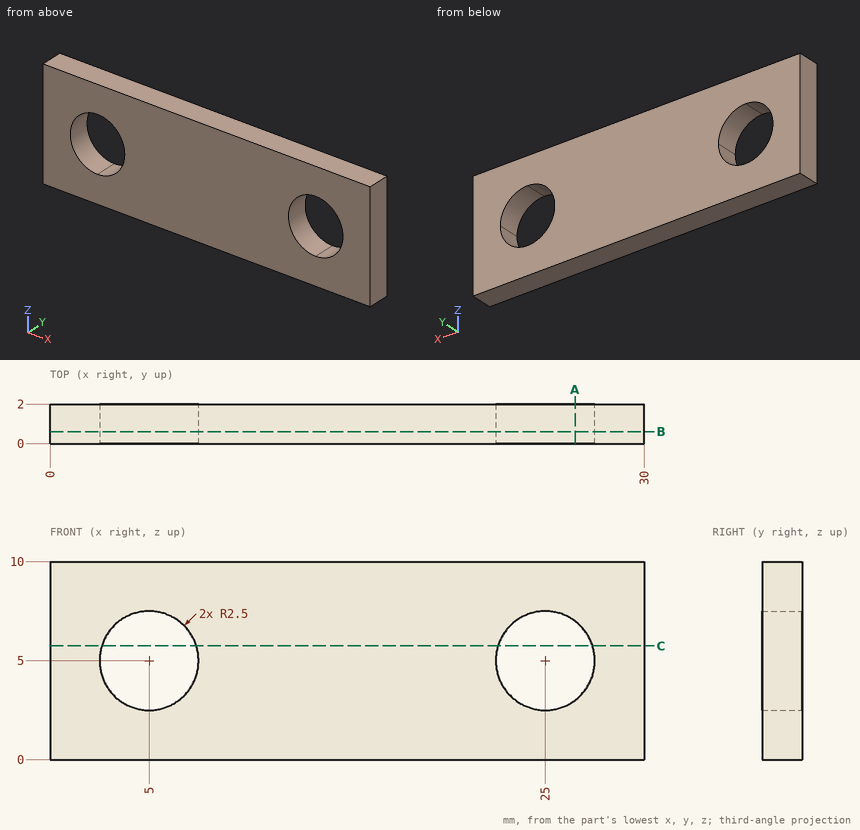
Answer from the drawing. Dimensions are ordinates in mm from the lowest x, y and z of the part. Give positions to 0.01 mm unless a question says otherwise; leave off trailing zeros. Loops run counter-clockwise (first coordinate to the right, second up) from the corner with the lowest first, then second, coordinate; pieces in that order, holes last.
Item 1: The part is cut by section A-A (x = 26.5). Write down the section's boundary in (y, z).
Item 2: The part is cut by section B-B (y = 0.6). Write down the section's boundary in (x, z).
Item 3: Find the intervals of material crossed by line 1 along X through (y, z) = (1.5, 6); line 2 along X through (y, z) = (0.25, 3.5); line 3 along Z through (x, y) = (4.5, 0.8), in increasing order.
Item 4: The part is cut by section C-C (z = 5.75). Write down the section's boundary in (x, y), and give its area (3 significant figures).
Taken from the geometry:
1. outline: (0, 0) - (2, 0) - (2, 3) - (0, 3) - close; (0, 7) - (2, 7) - (2, 10) - (0, 10) - close
2. outline: (0, 0) - (30, 0) - (30, 10) - (0, 10) - close; hole circle Ø5 at (5, 5); hole circle Ø5 at (25, 5)
3. line 1: x = 0 to 2.71, 7.29 to 22.71, 27.29 to 30
3. line 2: x = 0 to 3, 7 to 23, 27 to 30
3. line 3: z = 0 to 2.55, 7.45 to 10
4. outline: (0, 0) - (2.62, 0) - (2.62, 2) - (0, 2) - close; (7.38, 0) - (22.62, 0) - (22.62, 2) - (7.38, 2) - close; (27.38, 0) - (30, 0) - (30, 2) - (27.38, 2) - close
4. area: 40.9 mm2
